CAD build for the part. Positions are in the model's coordinates, mm. A direction names the side the tool comes from. Give positions to 0.01 mm unless a question says otherwise; leave off trailing zeros. Write each loop counter-clockwise with the first axis right and the second up, starting at its lowest first coordinate (ties: lowest second). Pieces come first, ordered by that corner, then holes. Notation, with made-up numbers: (76.5, -6) - (98.5, -6) arc R26 ccw to (98.5, 17) - close; hole circle Ø6 at (69.25, -28.5). An arc over 180 degrees is marked (long way). Put each result on its own line as item: value. Start each with the question number.
1. Cut at B-B on y = -14.75. List the corners of the cut face in (x, z).
2. Cut at A-A on x = 3. List the corners of the cut face in (y, z), and give its area (3 significant figures).
3. Wall check: line 1 (X direction, y = -8, z = -0.25); line 2 (Y direction, x = -7.75, z = 4.25); line 3 (Z direction, x = 6, y = -6.75). Give the ranges that are in metal, low to high.
4. Cut at D-D on y = -18.25. List the corners of the cut face in (x, z), and give its area (3 significant figures).
5. Drop flat-ended pins along their axis: pin 1 (10 mm diameter, centred on x = 1.5, y = -17, fed in from +Z); pin 2 (10 mm diameter, centred on x = -2.5, y = -11, fed in from +Z); pin 3 (1.1 mm diameter, centred on x = -1, z = 3, fed in from +Y); pin 4 (4 mm diameter, centred on y = -15.5, z = 12.5, fed in from +X). Give the stop position or say it passes through.
6. Cut at C-C on x = -4. List the corners of the cut face in (y, z), and give its area (3 significant figures).
7. Tool access for faces 5 (the flat face through (1, -20.421, 3)), 6 (the cylindrical face through (9.27, -8.55, 13.96)), 7 (the cylindrical face through (-4.94, -7.17, -0.74)), 8 (the flat face through (1.111, -10.012, 12.935)): list every direction of +Z, -Z, +X, -X, +Y, -Y with a clear straight run to the whole face (end or side of a thin tool).
8. Mould opens along Z. For faces 1 (the cylindrical face through (0.88, -21.675, 5.355)), 2 (the cylindrical face through (7.06, -7.17, -0.74)), 3 (the cylindrical face through (-7.23, -8.61, 13.92)), 4 (the flat face through (0.88, -13.973, 9.233)) say: +Z half, -Z half, draft (parallel to the pull), parting line (faces both ways), or undercut.
from build123d import *

# Parameters (mm, degrees)
SKETCH1_W                    = 20
SKETCH1_H                    = 22
BASE_FLANGE1_DEPTH           = 1.5
EDGE_FLANGE1_STRIP_W         = 7.4732
EDGE_FLANGE1_STRIP_H         = 1.5
EDGE_FLANGE1_STRIP_CUT_DEPTH = 20
EDGE_FLANGE1_DEPTH           = 20
EDGE_FLANGE2_START           = -8.98015873
EDGE_FLANGE2_DEPTH           = 20
EDGE_FLANGE2_2_DEPTH         = 20
CUT_EXTRUDE1_DEPTH           = 10
CHAMFER1_SIZE                = 1
CHAMFER2_SIZE                = 1


# Read off the part's stored shape, not the designer's step: Edge-Flange2
# Sheet-metal steps are written as plain solids
with BuildPart() as part:
    # Sketch1 → Base-Flange1 (new body)
    with BuildSketch(Plane.XY):
        with Locations((1.01984127, -10.920634921)):
            Rectangle(SKETCH1_W, SKETCH1_H)
        with BuildLine():
            Line((-6.73015873, -8.920634921), (-6.73015873, -16.920634921))
            ThreePointArc((-6.73015873, -16.920634921), (-4.98015873, -18.670634921), (-3.23015873, -16.920634921))
            Line((-3.23015873, -16.920634921), (-3.23015873, -8.920634921))
            ThreePointArc((-3.23015873, -8.920634921), (-4.98015873, -7.170634921), (-6.73015873, -8.920634921))
        make_face(mode=Mode.SUBTRACT)
        with BuildLine():
            Line((5.26984127, -8.920634921), (5.26984127, -16.920634921))
            ThreePointArc((5.26984127, -16.920634921), (7.01984127, -18.670634921), (8.76984127, -16.920634921))
            Line((8.76984127, -16.920634921), (8.76984127, -8.920634921))
            ThreePointArc((8.76984127, -8.920634921), (7.01984127, -7.170634921), (5.26984127, -8.920634921))
        make_face(mode=Mode.SUBTRACT)
    extrude(amount=-BASE_FLANGE1_DEPTH)

    # Edge-Flange1 strip (across the edge) → Edge-Flange1 strip cut (cut)
    with BuildSketch(Plane(origin=(-8.98015873, -21.920634921, 0), x_dir=(0, 1, 0), z_dir=(1, 0, 0))):
        with Locations((-1.5, -0.75)):
            Rectangle(EDGE_FLANGE1_STRIP_W, EDGE_FLANGE1_STRIP_H)
    extrude(amount=EDGE_FLANGE1_STRIP_CUT_DEPTH, mode=Mode.SUBTRACT)

    # Edge-Flange1 section (across the edge) → Edge-Flange1 (add)
    with BuildSketch(Plane(origin=(-8.98015873, -21.920634921, 0), x_dir=(0, 1, 0), z_dir=(1, 0, 0))):
        with BuildLine():
            Line((0, 0.7366), (0, 6.55))
            Line((0, 6.55), (1.5, 6.55))
            Line((1.5, 6.55), (1.5, 0.7366))
            ThreePointArc((1.5, 0.7366), (1.715745145, 0.215745145), (2.2366, 0))
            Line((2.2366, 0), (2.2366, -1.5))
            ThreePointArc((2.2366, -1.5), (0.655084973, -0.844915027), (0, 0.7366))
        make_face()
    extrude(amount=EDGE_FLANGE1_DEPTH)

    # Edge-Flange2 outline → Edge-Flange2 (cut)
    with BuildSketch(Plane.YZ.offset(EDGE_FLANGE2_START)):
        with BuildLine():
            ThreePointArc((-21.920634921, 4.335388427), (-21.66792335, 5.368135376), (-20.966895978, 6.16750389))
            Line((-20.966895978, 6.16750389), (-20.420634921, 6.55))
            Line((-20.420634921, 6.55), (-21.920634921, 6.55))
            Line((-21.920634921, 6.55), (-21.920634921, 4.335388427))
        make_face()
    extrude(amount=EDGE_FLANGE2_DEPTH, mode=Mode.SUBTRACT)

    # Edge-Flange2 2 outline → Edge-Flange2 2 (add)
    with BuildSketch(Plane.YZ.offset(EDGE_FLANGE2_START)):
        with BuildLine():
            Line((-4.906846961, 17.412871276), (-20.420634921, 6.55))
            Line((-20.420634921, 6.55), (-20.420634921, 4.335388427))
            ThreePointArc((-20.420634921, 4.335388427), (-20.3374071, 4.675512455), (-20.106531324, 4.938775823))
            Line((-20.106531324, 4.938775823), (-4.046482306, 16.184143209))
            Line((-4.046482306, 16.184143209), (-4.906846961, 17.412871276))
        make_face()
    extrude(amount=EDGE_FLANGE2_2_DEPTH)

    # Sketch12 → Cut-Extrude1 (cut)
    with BuildSketch(Plane(origin=(0, -9.795676552, 13.989675943), x_dir=(1, 0, 0), z_dir=(0, -0.5735764363510533, 0.8191520442889869))):
        with BuildLine():
            Line((7.51984127, -0.781841066), (-5.48015873, -0.781841066))
            ThreePointArc((-5.48015873, -0.781841066), (-7.23015873, 0.968158934), (-5.48015873, 2.718158934))
            Line((-5.48015873, 2.718158934), (7.51984127, 2.718158934))
            ThreePointArc((7.51984127, 2.718158934), (9.26984127, 0.968158934), (7.51984127, -0.781841066))
        make_face()
    extrude(amount=-CUT_EXTRUDE1_DEPTH, mode=Mode.SUBTRACT)

    # Chamfer1
    chamfer1_edges = [part.edges().sort_by_distance(p)[0] for p in [
        (11.01984127, 0.079365079, -0.75),
    ]]
    chamfer(chamfer1_edges, length=CHAMFER1_SIZE)

    # Chamfer2
    chamfer2_edges = [part.edges().sort_by_distance(p)[0] for p in [
        (-8.98015873, 0.079365079, -0.75),
        (-8.98015873, -4.476664634, 16.798507243),
        (11.01984127, -4.476664634, 16.798507243),
    ]]
    chamfer(chamfer2_edges, length=CHAMFER2_SIZE)


solid = part.part
Report:
1. outline: (-8.98, -1.5) - (-6.73, -1.5) - (-6.73, 0) - (-8.98, 0) - close; (-8.98, 8.69) - (11.02, 8.69) - (11.02, 10.52) - (-8.98, 10.52) - close; (-3.23, -1.5) - (5.27, -1.5) - (5.27, 0) - (-3.23, 0) - close; (8.77, -1.5) - (11.02, -1.5) - (11.02, 0) - (8.77, 0) - close
2. outline: (-21.92, 0.74) arc R2.24 ccw to (-19.68, -1.5) - (0.08, -1.5) - (0.08, 0) - (-19.68, 0) arc R0.74 cw to (-20.42, 0.74) - (-20.42, 4.34) arc R0.74 cw to (-20.11, 4.94) - (-9.58, 12.31) - (-10.44, 13.54) - (-20.97, 6.17) arc R2.24 ccw to (-21.92, 4.34) - close; (-7.57, 15.55) - (-6.71, 14.32) - (-4.05, 16.18) - (-4.91, 17.41) - close
2. area: 64.8 mm²
3. line 1: x = -8.98 to -6.47, -3.49 to 5.53, 8.51 to 11.02
3. line 2: y = -21.92 to -20.42
3. line 3: z = -1.5 to 0, 14.38 to 16.12
4. outline: (-8.98, -1.5) - (-6.12, -1.5) - (-6.12, 0) - (-8.98, 0) - close; (-8.98, 6.24) - (11.02, 6.24) - (11.02, 8.07) - (-8.98, 8.07) - close; (-3.84, -1.5) - (5.88, -1.5) - (5.88, 0) - (-3.84, 0) - close; (8.16, -1.5) - (11.02, -1.5) - (11.02, 0) - (8.16, 0) - close
4. area: 59.8 mm²
5. pin 1: stops at z = 12.45
5. pin 2: stops at z = 16.65
5. pin 3: stops at y = -20.42
5. pin 4: passes through
6. outline: (-21.92, 0.74) arc R2.24 ccw to (-19.68, -1.5) - (-18.37, -1.5) - (-18.37, 0) - (-19.68, 0) arc R0.74 cw to (-20.42, 0.74) - (-20.42, 4.34) arc R0.74 cw to (-20.11, 4.94) - (-9.58, 12.31) - (-10.44, 13.54) - (-20.97, 6.17) arc R2.24 ccw to (-21.92, 4.34) - close; (-7.57, 15.55) - (-6.71, 14.32) - (-4.05, 16.18) - (-4.91, 17.41) - close; (-7.47, -1.5) - (0.08, -1.5) - (0.08, 0) - (-7.47, 0) - close
6. area: 48.5 mm²
7. face 5: +X, -X, +Y
7. face 6: none
7. face 7: -Z
7. face 8: +Z, +Y
8. face 1: +Z half
8. face 2: draft
8. face 3: undercut
8. face 4: undercut
